Source: CAD feature listing. Evaluate the final solid. Frame: model axes, mm. A direction names the side the tool comes from. Round coordinates to 2 decimals unless told otherwise and drop trailing zeros. Order: outer loops, then holes, each group sorted by start corner. A loop starts at its lowest first (then second) coordinate and runs counter-clockwise, first axis right, second up. Notation, with made-up numbers: (41, -22) - (52, -22) arc R19 ccw to (52, -8) - close; hole circle Ø6 at (41, 50). An arc over 180 degrees is marked (long way). Use one line per item in the form item = value. Start each with the question number.
Q1. Ray query, line 1 (Y direction, x = 0, z = 41); line 2 (Y direction, x = 14.5, z = 44.5); line 3 (X direction, y = -16, z = 1). Return the intervals inside material, ascending. Write a range as [from, to].
Q2. Cut plane D-D, the plane y = -10.5. Return the cut outline in (x, z).
Q3. Draft query along X for faces 1 (the flat face through (5, -27, 0)), 2 (the cylindrical face through (-15.759, 15.707, -0.714)). Return one class per face: released by +X, released by -X, zero draft, split by the parting line, or undercut.
Q4. Cut plane A-A, the plane y = 0. Return the cut outline in (x, z), and give its area (3 significant figures).
Q5. Cut plane C-C, the plane z = 4. Give the number of separate pieces and of enclosed holes in the cut face, and give its area (3 significant figures).
Q6. Set-up query: faces 3 (the flat face through (0, -25.6, 32)), 4 (the flat face through (14.399, -18.076, 31.61)). Return all of +Z, -Z, +X, -X, +Y, -Y with unobstructed straight access to the full face (end or side cutting, diameter ignored); none if empty.
Q7. Pin query (flat end, axial travel): pin 1 Ø2 at (y, z) = (-24, 42.5) entering from +X; pin 2 Ø10 at (x, z) = (-10, 23) entering from +Y; pin 3 Ø6 at (x, z) = (12, 40) entering from +Y. Return the tip coordinate at first contact, or that it passes through.
from build123d import *

# Parameters (mm, degrees)
F0_R     = 27
F0_R_2   = 19.25
F1_DEPTH = 64
F2_R     = 32.5
F2_R_2   = 19.25
F3_DEPTH = 1.7
F4_W     = 5.2
F4_H     = 5.2
F5_DEPTH = 65.701
F6_R     = 24
F6_R_2   = 22.25
F7_DEPTH = 2


with BuildPart() as f1:
    # F0 (on Top) → F1 (new body)
    with BuildSketch(Plane.XY):
        Circle(F0_R)
        Circle(F0_R_2, mode=Mode.SUBTRACT)
    extrude(amount=F1_DEPTH)

    # F2 (on face) → F3 (join)
    with BuildSketch(Plane(origin=(0, 0, 0), x_dir=(1, 0, 0), z_dir=(0, 0, -1))):
        Circle(F2_R)
        Circle(F2_R_2, mode=Mode.SUBTRACT)
    extrude(amount=F3_DEPTH)

    # F4 (on face) → F5 (cut, through all)
    with BuildSketch(Plane.XY.offset(64)):
        with Locations((0, -23)):
            Rectangle(F4_W, F4_H)
        Polygon((16.263456, -12.586501), (12.586501, -16.263456), (16.263456, -19.940411), (19.940411, -16.263456), align=None)
        with Locations((23, 0)):
            Rectangle(F4_W, F4_H)
        Polygon((12.586501, 16.263456), (16.263456, 12.586501), (19.940411, 16.263456), (16.263456, 19.940411), align=None)
        with Locations((0, 23)):
            Rectangle(F4_W, F4_H)
        Polygon((-16.263456, 12.586501), (-12.586501, 16.263456), (-16.263456, 19.940411), (-19.940411, 16.263456), align=None)
        with Locations((-23, 0)):
            Rectangle(F4_W, F4_H)
        Polygon((-12.586501, -16.263456), (-16.263456, -12.586501), (-19.940411, -16.263456), (-16.263456, -19.940411), align=None)
    extrude(amount=-F5_DEPTH, mode=Mode.SUBTRACT)

    # F6 (on face) → F7 (join)
    with BuildSketch(Plane(origin=(0, 0, -1.7), x_dir=(1, 0, 0), z_dir=(0, 0, -1))):
        Circle(F6_R)
        Circle(F6_R_2, mode=Mode.SUBTRACT)
    extrude(amount=-F7_DEPTH)


solid = f1.part
Completed:
q1.line_1 = [-27, -25.6], [-20.4, -19.25], [19.25, 20.4], [25.6, 27]
q1.line_2 = [-22.78, -18.18], [-14.35, -12.66], [12.66, 14.35], [18.18, 22.78]
q1.line_3 = [-21.75, -19.68], [-12.85, -10.7], [10.7, 12.85], [19.68, 21.75]
q2.outline = (-30.76, -1.7) - (-16.13, -1.7) - (-16.13, 64) - (-24.87, 64) - (-24.87, 0) - (-30.76, 0) - close; (16.13, -1.7) - (30.76, -1.7) - (30.76, 0) - (24.87, 0) - (24.87, 64) - (16.13, 64) - close
q3.face_1 = zero draft
q3.face_2 = undercut
q4.outline = (-32.5, -1.7) - (-25.6, -1.7) - (-25.6, 64) - (-27, 64) - (-27, 0) - (-32.5, 0) - close; (-24, -1.7) - (-22.25, -1.7) - (-22.25, 0.3) - (-24, 0.3) - close; (-20.4, -1.7) - (-19.25, -1.7) - (-19.25, 64) - (-20.4, 64) - close; (19.25, -1.7) - (20.4, -1.7) - (20.4, 64) - (19.25, 64) - close; (22.25, -1.7) - (24, -1.7) - (24, 0.3) - (22.25, 0.3) - close; (25.6, -1.7) - (32.5, -1.7) - (32.5, 0) - (27, 0) - (27, 64) - (25.6, 64) - close
q4.area = 361 mm2
q5.separate_pieces = 1
q5.enclosed_holes = 9
q5.area = 910 mm2
q6.face_3 = +Z, -Z
q6.face_4 = +Z
q7.pin_1 = 14.14
q7.pin_2 = 26.53
q7.pin_3 = 25.46
